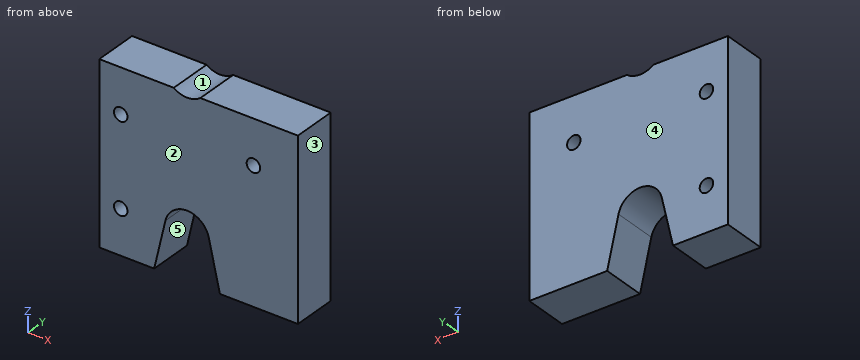
Autodesk Inventor part; units mm, degrees
ref_plane "YZ Plane" through (0, 0, 0) normal (1, 0, 0) x (0, 1, 0)
ref_plane "XZ Plane" through (0, 0, 0) normal (0, 1, 0) x (-1, 0, 0)
ref_plane "XY Plane" through (0, 0, 0) normal (0, 0, 1) x (1, 0, 0)
sketch "Sketch1" plane through (0, 0, 0) normal (0, 1, 0) x (-1, 0, 0)
  circle A0 centre (73.1106, 19.0179) radius 0.9652
  circle A1 centre (73.1106, 31.7179) radius 0.9652
  circle A2 centre (54.1114, 31.7179) radius 0.9652
  line L0 (58.8995, 12.6679) -> (60.5161, 19.7267)
  arc A3 (66.7058, 19.7267) -> (60.5161, 19.7267) centre (63.611, 19.0179) ccw
  line L1 (66.7058, 19.7267) -> (68.3224, 12.6679)
  arc A4 (61.706, 38.0679) -> (65.516, 38.0679) centre (63.611, 40.6079) ccw
  line L2 (79.486, 38.0679) -> (79.486, 12.6679) construction
  line L3 (47.736, 12.6679) -> (47.736, 38.0679)
  line L4 (47.736, 38.0679) -> (61.706, 38.0679)
  line L5 (65.516, 38.0679) -> (79.486, 38.0679) construction
  line L6 (79.486, 12.6679) -> (68.3224, 12.6679) construction
  line L7 (58.8995, 12.6679) -> (47.736, 12.6679)
  line L8 (76.184, 38.0679) -> (76.184, 12.6679)
  line L9 (65.516, 38.0679) -> (76.184, 38.0679)
  line L10 (68.3224, 12.6679) -> (76.184, 12.6679)
  point P0 (0, 0)
  dimension "d9" = 1.9304
  dimension "d10" = 25.4
  dimension "d11" = 31.75
  dimension "d14" = 18.9992
  dimension "d15" = 6.3754
  dimension "d16" = 15.875
  dimension "d17" = 15.875
  dimension "d18" = 28.448
extrude "Extrusion1" add sketch "Sketch1" along normal blind 6.35
sketch "Sketch3" plane through (0, 0, 0) normal (0, -1, 0) x (1, 0, 0)
  arc A0 (-60.5161, 19.7267) -> (-66.7058, 19.7267) centre (-63.611, 19.0179) ccw
  line L0 (-58.8995, 12.6679) -> (-60.5161, 19.7267)
  line L1 (-47.736, 12.6679) -> (-58.8995, 12.6679)
  line L2 (-47.736, 38.0679) -> (-47.736, 12.6679)
  line L3 (-61.706, 38.0679) -> (-47.736, 38.0679)
  arc A1 (-65.516, 38.0679) -> (-61.706, 38.0679) centre (-63.611, 40.6079) ccw
  line L4 (-76.184, 38.0679) -> (-65.516, 38.0679)
  line L5 (-76.184, 12.6679) -> (-76.184, 38.0679)
  line L6 (-68.3224, 12.6679) -> (-76.184, 12.6679)
  line L7 (-66.7058, 19.7267) -> (-68.3224, 12.6679)
  circle A2 centre (-54.1114, 31.7179) radius 0.9652
  circle A3 centre (-73.1106, 31.7179) radius 0.9652
  circle A4 centre (-73.1106, 19.0179) radius 0.9652
  point P0 (0, 0)
properties part number "delrin for sides" material "UHMW, White"
Check sheet for the modelled part. Datum: model origin and axes. Units: mm. Face numbers are marked on the shaded views. A direction names the side the tool comes from. Round coordinates to 2 decimals unless told otherwise and drop trailing zeros. Loops run counter-clockwise (first coordinate to the right, second up) from the corner with the lowest first, then second, coordinate; pieces in that order, holes last. Notation, with made-up numbers: (-21.5, -8) - (36.5, -8) arc R26 ccw to (36.5, 17) - close; hole circle Ø6 at (62, 50.5). An arc over 180 degrees is marked (long way). Answer as a JSON object with one key per item and string values. Group by question number.
Q1. Sectioned sample at B-B, the plane z = 21.5. Enter the section's corners in (x, y).
Q2. Mould release check, pull along X, two halves, no side actions. Record for the marked faces 1, 2 and 3: released by +X, released by -X, zero draft, split by the parting line, or undercut.
Q3. Gauge pin test, flat end, axial feed: P1, Ø1, axis at x = -62.5, y = 5, coming from the +Z side. Record the tip position at first contact, or that the pin passes through.
Q4. Sectioned sample at D-D, the plane x = -62.25. Enter the section's corners in (y, z), plus the area to 3 significant figures.
Q5. Set-up check for the marked faces 4 and 5: record each of +Z, -Z, +X, -X, +Y, -Y from which the full face is reachable in a straight line by a thin tool's end or side.
Q6. Sectioned sample at C-C, the plane y = 5.5. Count the separate pieces of the cut face and the enclosed holes in it, plus the area to 3 significant figures.
Q7. Scan lines: line 1 along X through (y, z) = (2.5, 19); line 2 along X through (y, z) = (0.75, 18.5); line 3 along X through (y, z) = (1.5, 15.75). Record each from-to range of solid material in increasing order. Write a range as [from, to].
Q8. Sectioned sample at A-A, the plane z = 32.25. Enter the section's corners in (x, y).
Solution:
{
 "1": {"outline": "(-76.18, 0) - (-65.59, 0) - (-65.59, 6.35) - (-76.18, 6.35) - close; (-61.63, 0) - (-47.74, 0) - (-47.74, 6.35) - (-61.63, 6.35) - close"},
 "2": {"face 1": "undercut", "face 2": "zero draft", "face 3": "released by +X"},
 "3": {"P1": "stops at z = 37.87"},
 "4": {"outline": "(0, 21.89) - (6.35, 21.89) - (6.35, 37.74) - (0, 37.74) - close", "area": "101 mm²"},
 "5": {"face 4": "+Z, -Z, +X, -X, +Y", "face 5": "-Z, +Y, -Y"},
 "6": {"separate pieces": "1", "enclosed holes": "3", "area": "646 mm²"},
 "7": {"line 1": "x = [-76.18, -74.08], [-72.15, -66.87], [-60.35, -47.74]", "line 2": "x = [-76.18, -73.93], [-72.3, -66.99], [-60.24, -47.74]", "line 3": "x = [-76.18, -67.62], [-59.61, -47.74]"},
 "8": {"outline": "(-76.18, 0) - (-73.92, 0) - (-73.92, 6.35) - (-76.18, 6.35) - close; (-72.31, 0) - (-54.92, 0) - (-54.92, 6.35) - (-72.31, 6.35) - close; (-53.31, 0) - (-47.74, 0) - (-47.74, 6.35) - (-53.31, 6.35) - close"}
}
